The drawing under review shows one solid part. Ordinate dimensions are in mm from its lowest x, y, z. Round coordinates to 2 decimals unless told otherwise and drop trailing zeros. Order: outer loops, then holes, each group sorted by start corner. A loop starts at its lowest first (then second) coordinate and runs counter-clockwise, first axis right, second up. Notation, with made-up numbers: M 84,68.25 L 137,68.25 A13 ccw 137,81.25 Z; hole C 52,28.5 d6. An arc over 180 degrees is marked long. Answer as a JSON object with one key per item and string values. Group by question number.
1. Mouldability with a two-part tool opening along X and no side actions: class the marked faces 1 and 2 as released by +X, released by -X, zero draft, split by the parting line, or undercut.
2. Clearance check with flat-ended pins moving along their axes: P1, Ø2, axis at x = 17.5, y = 2.5, coming from the -Z side; P2, Ø1, axis at y = 4.5, z = 48.5, coming from the +X side; P3, Ø4.5, axis at x = 88, z = 88, coming from the +Y side. State where each tip first meets the part, or that it passes through.
3. To check wall thickness, follow probe 1 along X at (y, z) = (3, 89) (1 decimal); probe 2 along X at (y, z) = (8.3, 53); probe 3 along Y at (x, z) = (86.5, 89). State the ranges of each line that lie inside material, in increasing order. Write a range as [from, to].
4. Add section B-B on z = 53. State the section outline as (x, y) points.
5. Add section A-A on x = 53. State the section outline as (y, z) points, and give its area (3 significant figures).
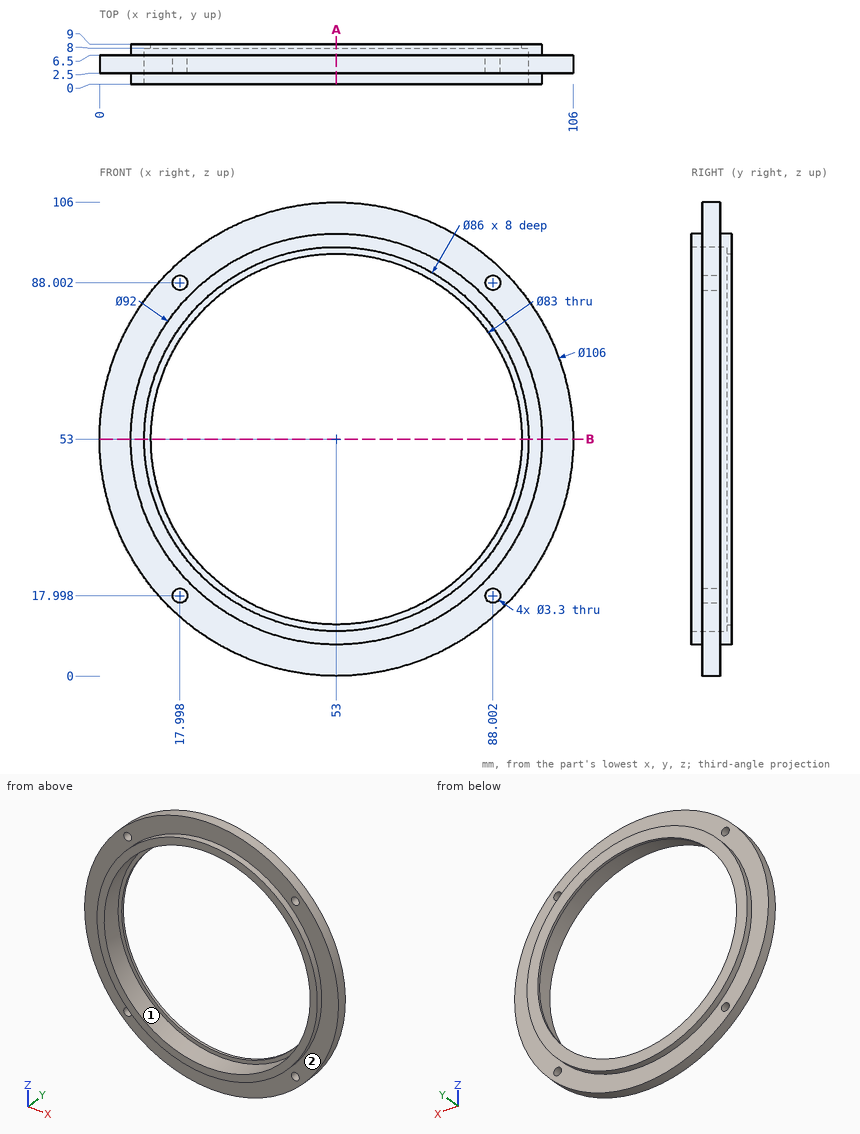
Recorded:
{
 "1": {"face 1": "undercut", "face 2": "zero draft"},
 "2": {"P1": "stops at z = 12.77", "P2": "stops at x = 105.85", "P3": "stops at y = 6.5"},
 "3": {"probe 1": "x = [14.1, 16.7], [19.3, 29.5], [76.5, 86.7], [89.3, 91.9]", "probe 2": "x = [7, 11.5], [94.5, 99]", "probe 3": "y = [2.5, 6.5]"},
 "4": {"outline": "M 0,2.5 L 7,2.5 L 7,0 L 10,0 L 10,8 L 11.5,8 L 11.5,9 L 7,9 L 7,6.5 L 0,6.5 Z; M 94.5,8 L 96,8 L 96,0 L 99,0 L 99,2.5 L 106,2.5 L 106,6.5 L 99,6.5 L 99,9 L 94.5,9 Z"},
 "5": {"outline": "M 0,7 L 2.5,7 L 2.5,0 L 6.5,0 L 6.5,7 L 9,7 L 9,11.5 L 8,11.5 L 8,10 L 0,10 Z; M 0,96 L 8,96 L 8,94.5 L 9,94.5 L 9,99 L 6.5,99 L 6.5,106 L 2.5,106 L 2.5,99 L 0,99 Z", "area": "113 mm²"}
}
